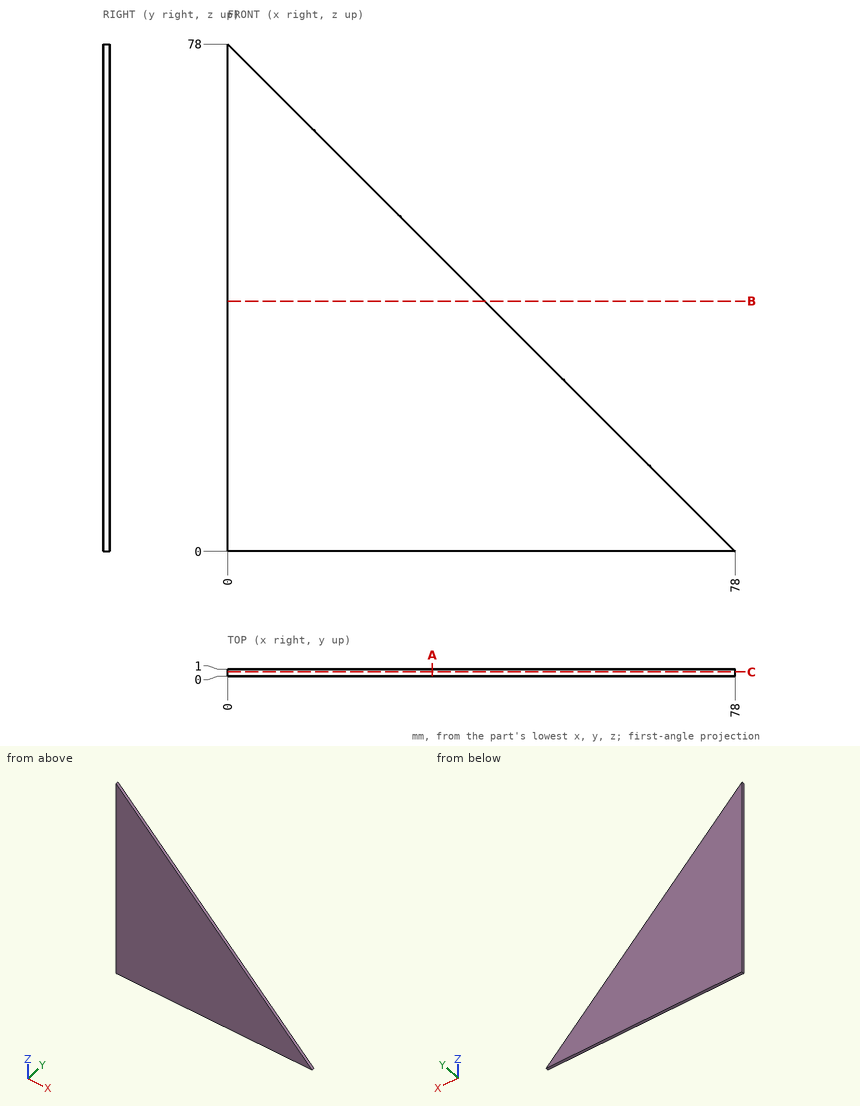
Geometry: see drawing. Coordinates: mm, zero at the bounding-box minimum. Round coordinates to 2 decimals unless told otherwise and drop trailing zeros. Loops run counter-clockwise (first coordinate to the right, second up) from the corner with the lowest first, then second, coordinate; pieces in that order, holes last. Notation, with made-up numbers: M -37,-26 L 10,-26 A13 cw 10,-14 Z; hole C 70.5,28 d9. An arc over 180 degrees is marked long. Use a Markdown table: item, result. Add a question column.
1. Contact query for a flat-ended pin moving along its axis: pin 1 (5 mm diameter, centred on x = 41, z = 21, fed in from -Y). Output: stop coordinate, or through.
2. Cut plane C-C, the plane y = 0.65. Output: boundary loops of the cut face in (x, z), and give its area (3 significant figures).
3. Cut plane B-B, the plane z = 38.5. Output: boundary loops of the cut face in (x, y), and give its area (3 significant figures).
4. Cut plane A-A, the plane x = 31.5. Output: boundary loops of the cut face in (y, z), and give its area (3 significant figures).
5. Ray query, line 1 along X through (y, z) = (0.35, 31.5); line 2 along X through (y, z) = (0.8, 71.5); line 3 along Z through (x, y) = (24.5, 0.15). Return the intervals inside material, ascending. Write a range as [from, to].
Solution:
| question | item | result |
|---|---|---|
| 1 | pin 1 | stops at y = 0 |
| 2 | outline | M 0,0 L 78,0 L 0,78 Z |
| 2 | area | 3,040 mm2 |
| 3 | outline | M 0,0 L 39.5,0 L 39.5,1 L 0,1 Z |
| 3 | area | 39.5 mm2 |
| 4 | outline | M 0,0 L 1,0 L 1,46.5 L 0,46.5 Z |
| 4 | area | 46.5 mm2 |
| 5 | line 1 | x = [0, 46.5] |
| 5 | line 2 | x = [0, 6.5] |
| 5 | line 3 | z = [0, 53.5] |
